Check sheet for the modelled part. Datum: model origin and axes. Units: mm. A direction names the side the tool comes from. Give positions to 0.01 mm unless a question says otherwise; leave off trailing zeros. Loops run counter-clockwise (first coordinate to the right, second up) from the corner with the lowest first, then second, coordinate; pieces in that order, holes last. Notation, with made-up numbers: (30, 54) - (61, 54) arc R21 cw to (61, 61) - close; hole circle Ø1 at (73.25, 50.25). An arc over 180 degrees is marked (long way). Use one line per item in the form item = value.
from build123d import *

# Parameters (mm, degrees)
F1_DEPTH = 1.6


with BuildPart() as f1:
    # F0 (on Top) → F1 (new body)
    with BuildSketch(Plane.XY):
        with BuildLine():
            ThreePointArc((0, 2.4), (-1.697056, -1.697056), (2.4, 0))
            ThreePointArc((2.4, 0), (1.697056, 1.697056), (0, 2.4))
        make_face()
        with BuildLine():
            ThreePointArc((2, 14), (-1.414214, 15.414214), (0, 12))
            ThreePointArc((0, 12), (1.414214, 12.585786), (2, 14))
        make_face()
        with BuildLine():
            Line((-2.812876, 3.944275), (-3.183357, 0.325944))
            ThreePointArc((-3.183357, 0.325944), (0, -3.2), (3.183357, 0.325944))
            Line((3.183357, 0.325944), (2.812876, 3.944275))
            ThreePointArc((2.812876, 3.944275), (2.656846, 7), (2.812876, 10.055725))
            Line((2.812876, 10.055725), (3.183357, 13.674056))
            ThreePointArc((3.183357, 13.674056), (0, 17.2), (-3.183357, 13.674056))
            Line((-3.183357, 13.674056), (-2.812876, 10.055725))
            ThreePointArc((-2.812876, 10.055725), (-2.656846, 7), (-2.812876, 3.944275))
        make_face()
        with BuildLine():
            ThreePointArc((0, 2.4), (1.697056, 1.697056), (2.4, 0))
            ThreePointArc((2.4, 0), (-1.697056, -1.697056), (0, 2.4))
        make_face(mode=Mode.SUBTRACT)
        with BuildLine():
            ThreePointArc((2, 14), (1.414214, 12.585786), (0, 12))
            ThreePointArc((0, 12), (-1.414214, 15.414214), (2, 14))
        make_face(mode=Mode.SUBTRACT)
    extrude(amount=F1_DEPTH)


solid = f1.part
Item 1: Mould release check, pull along Y, two halves, no side actions. Record for faces 1 (the face through (2.996, 11.84, 0.789)), 2 (the face through (3, 2.1, 0.8)), 3 (the face through (0, 7, 1.6)): released by +Y, released by -Y, zero draft, split by the parting line, or undercut.
Answer block:
face_1 = undercut
face_2 = undercut
face_3 = zero draft
Item 2: Gauge pin test, flat ends, axial feed: P1, Ø1.5, axis at x = 0, y = 11.5, coming from the -Z side; P2, Ø3.5, axis at x = 0, y = 14, coming from the -Z side. Record the tip position at first contact, or that the pin passes through.
Answer block:
P1 = 0
P2 = through
Item 3: Section check D-D on x = 3. Record the boundary of the cut face in (y, z), then the cut area to 3 significant figures.
Answer block:
outline = (-1.11, 0) - (2.12, 0) - (2.12, 1.6) - (-1.11, 1.6) - close; (11.88, 0) - (15.11, 0) - (15.11, 1.6) - (11.88, 1.6) - close
area = 10.3 mm2
Item 4: Section check A-A on x = 1.5. Record the boundary of the cut face in (y, z), then the cut area to 3 significant figures.
Answer block:
outline = (-2.83, 0) - (-1.87, 0) - (-1.87, 1.6) - (-2.83, 1.6) - close; (1.87, 0) - (12.68, 0) - (12.68, 1.6) - (1.87, 1.6) - close; (15.32, 0) - (16.83, 0) - (16.83, 1.6) - (15.32, 1.6) - close
area = 21.2 mm2
Item 5: Access from +Z, -Z, +X, -X, +Y, -Y to the whole of each face (thin tool, end or side, straight path). Record for faces 4 (the face through (2.657, 6.957, 0.789)), 5 (the face through (-2.996, 2.16, 0.789)).
Answer block:
face_4 = +Z, -Z, +X
face_5 = +Z, -Z, -X
Item 6: Section check B-B on y = 12.5. Record the boundary of the cut face in (x, z).
Answer block:
outline = (-3.06, 0) - (-1.32, 0) - (-1.32, 1.6) - (-3.06, 1.6) - close; (1.32, 0) - (3.06, 0) - (3.06, 1.6) - (1.32, 1.6) - close
Item 7: Section check C-C on z = 1.15. Record the boundary of the cut face in (x, y), then the cut area to 3 significant figures.
Answer block:
outline = (-3.18, 0.33) arc R3.2 ccw (long way) to (3.18, 0.33) - (2.81, 3.94) arc R30 cw to (2.81, 10.06) - (3.18, 13.67) arc R3.2 ccw (long way) to (-3.18, 13.67) - (-2.81, 10.06) arc R30 cw to (-2.81, 3.94) - close; hole (0, 2.4) arc R2.4 ccw (long way) to (2.4, 0) arc R2.4 ccw to start; hole (0, 12) arc R2 ccw to (2, 14) arc R2 ccw (long way) to start
area = 82.2 mm2
Item 8: Thickness scan on L1, parallel to Y at x = 0.5, z = 0.1; L2, parallel to Y at x = 0.75, z = 1.3; L3, parallel to Y at x = -2.5, z = 0.2. Record the ranges inside material, lowest first.
Answer block:
L1 = -3.16 to -2.35, 2.35 to 12.06, 15.94 to 17.16
L2 = -3.11 to -2.28, 2.28 to 12.15, 15.85 to 17.11
L3 = -2 to 16
